For this review, take the finished solid that the model builds, in its own axes (mm). A direction names the side the tool comes from. Coordinates: 2 decimals unless noted, no trailing zeros. Write each loop counter-clockwise with the first axis right and the second up, starting at its lowest first coordinate (ties: lowest second). Pieces come first, ordered by that corner, then holes.
```python
from build123d import *

# Parameters (mm, degrees)
BOSS_EXTRUDE1_DEPTH = 18.8
SKETCH2_R           = 1.5
CUT_EXTRUDE1_DEPTH  = 168.8
FILLET1_R           = 1
FILLET2_R           = 1


with BuildPart() as part:
    # Sketch1 → Boss-Extrude1 (new body)
    with BuildSketch(Plane.XY):
        with BuildLine():
            Line((53, 10), (40, 10))
            Line((40, 10), (40, -20))
            Line((40, -20), (34.641016151, -20))
            ThreePointArc((34.641016151, -20), (0, -37.877855496), (-34.641016151, -20))
            Line((-34.641016151, -20), (-40, -20))
            Line((-40, -20), (-40, 10))
            Line((-40, 10), (-53, 10))
            Line((-53, 10), (-53, -20))
            Line((-53, -20), (-55, -20))
            Line((-55, -20), (-55, -23))
            ThreePointArc((-55, -23), (-54.414213562, -24.414213562), (-53, -25))
            Line((-53, -25), (-41.872771696, -25))
            ThreePointArc((-41.872771696, -25), (-37.918765594, -25.814912317), (-34.609193147, -28.12683285))
            ThreePointArc((-34.609193147, -28.12683285), (0, -43.025434322), (34.609193147, -28.12683285))
            ThreePointArc((34.609193147, -28.12683285), (37.918765594, -25.814912317), (41.872771696, -25))
            Line((41.872771696, -25), (53, -25))
            ThreePointArc((53, -25), (54.414213562, -24.414213562), (55, -23))
            Line((55, -23), (55, -20))
            Line((55, -20), (53, -20))
            Line((53, -20), (53, 10))
        make_face()
    extrude(amount=BOSS_EXTRUDE1_DEPTH)

    # Sketch2 → Cut-Extrude1 (cut)
    with BuildSketch(Plane.ZY.offset(53)):
        with Locations((9.4, -5)):
            Circle(SKETCH2_R)
        with Locations((9.4, 5)):
            Circle(SKETCH2_R)
        with Locations((9.4, 0)):
            Circle(SKETCH2_R)
        with Locations((9.4, -10)):
            Circle(SKETCH2_R)
    extrude(amount=-CUT_EXTRUDE1_DEPTH, mode=Mode.SUBTRACT)

    # Fillet1
    fillet1_edges = [part.edges().sort_by_distance(p)[0] for p in [
        (-40, -20, 9.4),
        (-34.641016151, -20, 9.4),
        (34.641016151, -20, 9.4),
        (40, -20, 9.4),
    ]]
    fillet(fillet1_edges, radius=FILLET1_R)

    # Fillet2
    fillet2_edges = [part.edges().sort_by_distance(p)[0] for p in [
        (-55, -20, 9.4),
        (-53, -20, 9.4),
        (-40, 10, 9.4),
        (-53, 10, 9.4),
        (55, -20, 9.4),
        (53, -20, 9.4),
        (53, 10, 9.4),
        (40, 10, 9.4),
    ]]
    fillet(fillet2_edges, radius=FILLET2_R - 0.0001)  # a hair under: the kernel refuses the full size


solid = part.part
```
Q1. Add section D-D (y = -39.5). State the section outline as (x, z) points, then the cut area to 3 significant figures.
Ans:
outline: (-17.99, 0) - (17.99, 0) - (17.99, 18.8) - (-17.99, 18.8) - close
area: 676 mm2
Q2. For probe 1 along Y at (x, z) = (-45.5, 9.4); probe 2 along X at (y, z) = (7, 3.5); probe 3 along X at (y, z) = (-21, 7.5), list the stretches that pass through material, from the lowest coordinate up.
Ans:
probe 1: y = -25 to -11.5, -8.5 to -6.5, -3.5 to -1.5, 1.5 to 3.5, 6.5 to 10
probe 2: x = -53 to -40, 40 to 53
probe 3: x = -55 to -33.91, 33.91 to 55
Q3. Clearance check with flat-ended pins moving along their axes: pin 1 Ø3 at (x, z) = (-37.5, 14) entering from +Y; pin 2 Ø4 at (y, z) = (-10, 9.4) entering from -X; pin 3 Ø1.8 at (y, z) = (-10, 9.4) entering from -X; pin 4 Ø5.5 at (y, z) = (-6.5, 10.5) entering from +X. State where each tip first meets the part, or that it passes through.
Ans:
pin 1: stops at y = -20
pin 2: stops at x = -53
pin 3: passes through
pin 4: stops at x = 53
Q4. Add section C-C (x = 37.5). State the section outline as (y, z) points, then the cut area to 3 significant figures.
Ans:
outline: (-26.01, 0) - (-20, 0) - (-20, 18.8) - (-26.01, 18.8) - close
area: 113 mm2
Q5. Add section A-A (y = 0). State the section outline as (x, z) points, then the cut area to 3 significant figures.
Ans:
outline: (-53, 0) - (-40, 0) - (-40, 7.9) - (-53, 7.9) - close; (-53, 10.9) - (-40, 10.9) - (-40, 18.8) - (-53, 18.8) - close; (40, 0) - (53, 0) - (53, 7.9) - (40, 7.9) - close; (40, 10.9) - (53, 10.9) - (53, 18.8) - (40, 18.8) - close
area: 411 mm2
Q6. Tool access review of faces 1 (the flat face through (-48, -25, 9)), 2 (the flat face through (47, -25, 9)), 3 (the flat face through (-40, -5, 7)), 4 (the cylindrical face through (-46.59, 5.07, 7.9)): name each direction out of +Z, -Z, +X, -X, +Y, -Y from which nothing blocks a thin tool from reaching the whole face with its end or side.
Ans:
face 1: +Z, -Z, -X, -Y
face 2: +Z, -Z, +X, -Y
face 3: +Z, -Z, +Y
face 4: +X, -X
Q7. Draft analysis for pull direction X (two halves, no side actions). For faces 5 (the cylindrical face through (0.56, -37.874, 9.268)), 6 (the cylindrical face through (-0.542, -43.022, 9.268)), 7 (the flat face through (-55, -22, 9)), 8 (the cylindrical face through (-46.6, -10.9, 8.2)), state which applies: +X half, -X half, draft (parallel to the pull), parting line (faces both ways), or undercut.
Ans:
face 5: undercut
face 6: parting line
face 7: -X half
face 8: draft
